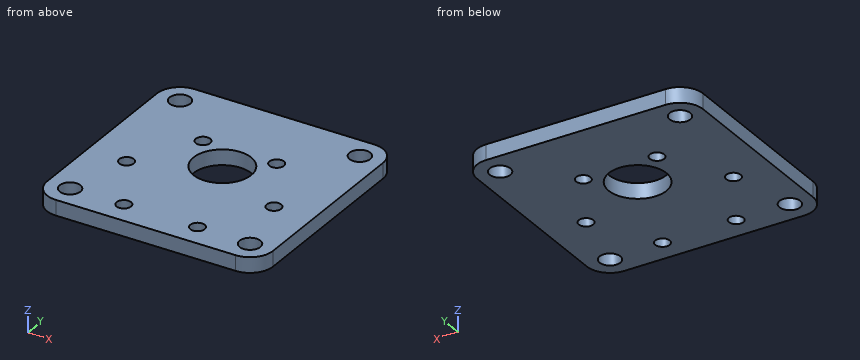
from build123d import *

# Parameters (mm, degrees)
F0_W     = 46.72538
F0_H     = 46.152003
F0_R     = 2.15265
F0_R_2   = 1.5
F0_R_3   = 5.969
F1_DEPTH = 3.175
F2_R     = 4.7625


with BuildPart() as f1:
    # F0 (on Top) → F1 (new body)
    with BuildSketch(Plane.XY):
        with Locations((0, 4.915002)):
            Rectangle(F0_W, F0_H)
        with Locations((-18.60019, -13.3985)):
            Circle(F0_R, mode=Mode.SUBTRACT)
        with Locations((-7.62, -13.198227)):
            Circle(F0_R_2, mode=Mode.SUBTRACT)
        with Locations((-15.24, 0)):
            Circle(F0_R_2, mode=Mode.SUBTRACT)
        with Locations((7.62, -13.198227)):
            Circle(F0_R_2, mode=Mode.SUBTRACT)
        with Locations((18.60019, -13.3985)):
            Circle(F0_R, mode=Mode.SUBTRACT)
        with Locations((15.24, 0)):
            Circle(F0_R_2, mode=Mode.SUBTRACT)
        with Locations((0, 7.366)):
            Circle(F0_R_3, mode=Mode.SUBTRACT)
        with Locations((-7.62, 13.198227)):
            Circle(F0_R_2, mode=Mode.SUBTRACT)
        with Locations((-18.60019, 23.228503)):
            Circle(F0_R, mode=Mode.SUBTRACT)
        with Locations((7.62, 13.198227)):
            Circle(F0_R_2, mode=Mode.SUBTRACT)
        with Locations((18.60019, 23.228503)):
            Circle(F0_R, mode=Mode.SUBTRACT)
    extrude(amount=F1_DEPTH)

    # F2
    f2_edges = [f1.edges().sort_by_distance(p)[0] for p in [
        (-23.36269, -18.161, 1.5875),
        (23.36269, -18.161, 1.5875),
        (23.36269, 27.991003, 1.5875),
        (-23.36269, 27.991003, 1.5875),
    ]]
    fillet(f2_edges, radius=F2_R)


solid = f1.part
Source: CAD feature listing. Evaluate the final solid. Frame: model axes, mm. Give positions to 0.01 mm unless a question says otherwise; leave off trailing zeros. Write each loop counter-clockwise with the first axis right and the second up, starting at its lowest first coordinate (ties: lowest second). Pieces come first, ordered by that corner, then holes. Notation, with made-up numbers: M 85,-19 L 112,-19 A14 ccw 112,-11 Z; hole C 22,-30.75 d4. An arc over 180 degrees is marked long. Return JSON: item names as keys, results as strings. Group by question number.
1) Cut plane C-C, the plane y = 5.5. Output: boundary loops of the cut face in (x, z) (3 decimals).
2) Ray query, L1, parallel to Y at x = -7.62, z = 0.9; L2, parallel to X at y = -1, z = 1.75; L3, parallel to Y at x = -17.5, z = 2.45. Return the intervals inside material, ascending.
3) Cut plane B-B, the plane x = -15.24. Output: boundary loops of the cut face in (y, z) (3 decimals), then the cut area to 3 significant figures.
4) Cut plane D-D, the plane y = 22.5. Output: boundary loops of the cut face in (x, z) (3 decimals).
5) Cut plane A-A, the plane x = -7.62. Output: boundary loops of the cut face in (y, z) (3 decimals).
Data:
{
 "1": {"outline": "M -23.363,0 L -5.67,0 L -5.67,3.175 L -23.363,3.175 Z; M 5.67,0 L 23.363,0 L 23.363,3.175 L 5.67,3.175 Z"},
 "2": {"L1": "y = -18.16 to -14.7, -11.7 to 11.7, 14.7 to 27.99", "L2": "x = -23.36 to -16.36, -14.12 to 14.12, 16.36 to 23.36", "L3": "y = -18.16 to -15.25, -11.55 to 21.38, 25.08 to 27.99"},
 "3": {"outline": "M -18.161,0 L -1.5,0 L -1.5,3.175 L -18.161,3.175 Z; M 1.5,0 L 27.991,0 L 27.991,3.175 L 1.5,3.175 Z", "area": "137 mm²"},
 "4": {"outline": "M -23.363,0 L -20.626,0 L -20.626,3.175 L -23.363,3.175 Z; M -16.575,0 L 16.575,0 L 16.575,3.175 L -16.575,3.175 Z; M 20.626,0 L 23.363,0 L 23.363,3.175 L 20.626,3.175 Z"},
 "5": {"outline": "M -18.161,0 L -14.698,0 L -14.698,3.175 L -18.161,3.175 Z; M -11.698,0 L 11.698,0 L 11.698,3.175 L -11.698,3.175 Z; M 14.698,0 L 27.991,0 L 27.991,3.175 L 14.698,3.175 Z"}
}
